Part model, mm, in its own coordinate system. Round coordinates to 2 decimals unless told otherwise and drop trailing zeros. Order: outer loops, then holes, each group sorted by start corner. A loop starts at its lowest first (then second) coordinate and runs counter-clockwise, first axis right, second up. Notation, with made-up numbers: (83, 56.25) -> (137, 56.25) arc R22 cw to (137, 92.25) -> close; hole circle Ø5 at (23, -23). An arc over 180 degrees is marked (long way). Return JSON: item names as keys, results as strings. Group by question number.
from build123d import *

# Parameters (mm, degrees)
BOSS_EXTRUDE2_DEPTH = 3.357


with BuildPart() as part:
    # Sketch1 → Boss-Extrude2 (new body)
    with BuildSketch(Plane(origin=(0, 0, 0), x_dir=(1, 0, 0), z_dir=(0, 1, 0))):
        with BuildLine():
            Line((35, 12.545008155), (85, 12.545008155))
            Line((85, 12.545008155), (85, -12.545008155))
            Line((85, -12.545008155), (35, -12.545008155))
            ThreePointArc((35, -12.545008155), (30.588727606, -8.870191163), (25, -7.555))
            Line((25, -7.555), (0, -7.57))
            Line((0, -7.57), (-25, -7.535))
            ThreePointArc((-25, -7.535), (-30.586810484, -8.844242442), (-35, -12.511710977))
            Line((-35, -12.511710977), (-85, -12.511710977))
            Line((-85, -12.511710977), (-85, 12.511710977))
            Line((-85, 12.511710977), (-35, 12.511710977))
            ThreePointArc((-35, 12.511710977), (-30.586810484, 8.844242442), (-25, 7.535))
            Line((-25, 7.535), (0, 7.57))
            Line((0, 7.57), (25, 7.555))
            ThreePointArc((25, 7.555), (30.588727606, 8.870191163), (35, 12.545008155))
        make_face()
    extrude(amount=BOSS_EXTRUDE2_DEPTH)


solid = part.part
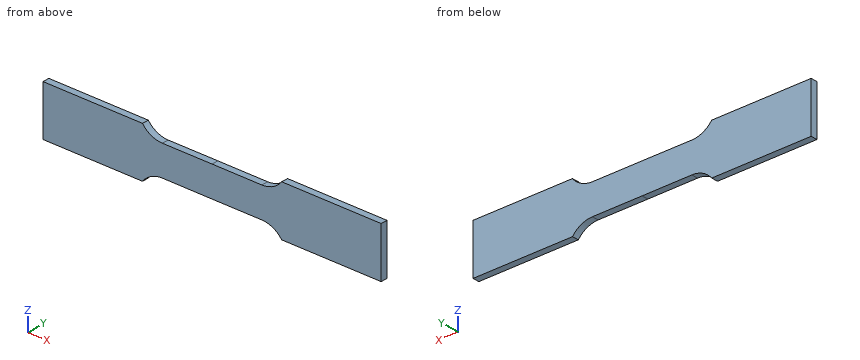
(1) Saw through at A-A, the plane z = -9.5. List the corners of the cut face in (x, y), and give its area (3 significant figures).
(2) Saw through at B-B, the plane y = 1.4. List the corners of the cut face in (x, z) (1 decimal), and give its area (3 significant figures).
(3) Probe L1, parallel to Z at x = 1.5, y = 1.05; L2, parallel to Z at x = -37, y = 2.9; L3, parallel to X at y = 1.25, z = 11.25. List the from-to ranges inside material, lowest first. Write a range as [from, to].
(4) Saw through at C-C, the plane x = 7. List the corners of the cut face in (y, z).
(5) Pin check, flat tips, straight feed: P1, Ø1, axis at x = -63, y = 1.5, coming from the +Z side; P2, Ø1.7, axis at x = -66, y = 1, coming from the -Z side. Stop position of each tip, or through.
Results are:
{
 "1": {"outline": "(-85, 0) -> (-31.75, 0) -> (-31.75, 3.36) -> (-85, 3.36) -> close; (31.7, 0) -> (85, 0) -> (85, 3.36) -> (31.7, 3.36) -> close", "area": "358 mm^2"},
 "2": {"outline": "(-85, -12.5) -> (-35, -12.5) arc R12.5 cw to (-25, -7.5) -> (0, -7.6) -> (25, -7.6) arc R12.5 cw to (35, -12.5) -> (85, -12.5) -> (85, 12.5) -> (35, 12.5) arc R12.5 cw to (25, 7.6) -> (0, 7.6) -> (-25, 7.5) arc R12.5 cw to (-35, 12.5) -> (-85, 12.5) -> close", "area": "3,620 mm^2"},
 "3": {"L1": "z = [-7.57, 7.57]", "L2": "z = [-12.51, 12.51]", "L3": "x = [-85, -33.91], [33.88, 85]"},
 "4": {"outline": "(0, -7.57) -> (3.36, -7.57) -> (3.36, 7.57) -> (0, 7.57) -> close"},
 "5": {"P1": "stops at z = 12.51", "P2": "stops at z = -12.51"}
}
